Work out the finished part from the listing and answer in its coordinate system (mm). Face numbers are marked on the shaded views. A direction names the side the tool comes from. Give positions to 0.01 mm unless a question says otherwise; leave off trailing zeros. Loops run counter-clockwise (first coordinate to the right, second up) from the corner with the lowest first, then second, coordinate; pieces in that order, holes last. Notation, with made-up numbers: (67.5, -18.5) - (82.5, -18.5) arc R24 cw to (82.5, 20.5) - close; hole circle Ø11 at (-39, -2.75). An arc over 180 degrees is marked (long way). One line per item, written item: value.
Autodesk Inventor part; units mm, degrees
ref_plane "YZ Plane" through (0, 0, 0) normal (1, 0, 0) x (0, 1, 0)
ref_plane "XZ Plane" through (0, 0, 0) normal (0, 1, 0) x (-1, 0, 0)
ref_plane "XY Plane" through (0, 0, 0) normal (0, 0, 1) x (1, 0, 0)
sketch "Sketch1" plane through (0, 0, 0) normal (0, 1, 0) x (-1, 0, 0)
  line L0 (0, 0) -> (200, 0)
  line L1 (200, 0) -> (200, -200)
  line L2 (200, -200) -> (0, -200)
  line L3 (0, -200) -> (0, 0)
  line L4 (198, -198) -> (198, -2)
  line L5 (198, -2) -> (2, -2)
  line L6 (2, -2) -> (2, -198)
  line L7 (2, -198) -> (198, -198)
  dimension "d0" = 200
  dimension "d1" = 200
  dimension "d2" = 2
extrude "Extrusion1" add sketch "Sketch1" against normal blind 65 contours L0 L1 L2 L3 | L7 L6 L5 L4
sketch "Sketch2" plane through (0, 0, 0) normal (0, 1, 0) x (1, 0, 0)
  line L0 (-198.5, 198.5) -> (-1.5, 198.5)
  line L1 (-1.5, 198.5) -> (-1.5, 1.5)
  line L2 (-1.5, 1.5) -> (-198.5, 1.5)
  line L3 (-198.5, 1.5) -> (-198.5, 198.5)
  line L4 (-200, 200) -> (-200, 0)
  line L5 (0, 200) -> (-200, 200)
  line L6 (-109.0225, 121.8048) -> (-59.0225, 121.8048)
  line L7 (-59.0225, 121.8048) -> (-59.0225, 76.8048)
  line L8 (-59.0225, 76.8048) -> (-109.0225, 76.8048)
  line L9 (-109.0225, 76.8048) -> (-109.0225, 121.8048)
  circle A0 centre (-100, 100) radius 4
  point P0 (0, 0)
  dimension "d5" = 197
  dimension "d6" = 197
  dimension "d7" = 1.5
  dimension "d8" = 1.5
  dimension "d37" = 50
  dimension "d38" = 45
  dimension "d39" = 8
extrude "Extrusion2" cut sketch "Sketch2" against normal blind 63 contours L0 L1 L2 L3 | L6 L7 L8 L9 | A0
sketch "Sketch3" plane through (-200, 0, 0) normal (0, 0, 1) x (1, 0, 0)
  line L0 (25, -35) -> (25, -65)
  line L1 (25, -65) -> (175, -65)
  line L2 (175, -65) -> (175, -35)
  line L3 (175, -35) -> (25, -35)
  line L4 (200, 0) -> (200, -65)
  line L5 (42.8625, -63) -> (47.625, -63)
  line L6 (198.5, -63) -> (1.5, -63)
  line L7 (200, -65) -> (0, -65)
  dimension "d11" = 150
  dimension "d12" = 30
  dimension "d13" = 25
  dimension "d14" = 0
  dimension "d36" = 0
extrude "Extrusion3" cut sketch "Sketch3" against normal blind 3
sketch "Sketch4" plane through (0, 0, -200) normal (0, 0, -1) x (-1, 0, 0)
  line L0 (40.0009, -61.5) -> (40.0009, -46.5)
  line L1 (0.0009, -46.5) -> (40.0009, -46.5)
  line L2 (40.0009, -61.5) -> (0.0009, -61.5)
  line L3 (0.0009, -61.5) -> (0.0009, -46.5)
  line L4 (0.0009, -46.5) -> (40.0009, -46.5)
  line L5 (40.0009, -46.5) -> (40.0009, -61.5)
  line L6 (200, -65) -> (0, -65)
  point P0 (48.3834, -59.8808)
  point P1 (40.0009, -54)
  point P2 (0.0009, -54)
  dimension "d27" = 40
  dimension "d28" = 15
  dimension "d29" = 3.5
extrude "Extrusion4" cut sketch "Sketch4" against normal blind 3
sketch "Sketch5" plane through (0, 0, 0) normal (1, 0, 0) x (0, 0, -1)
  line L0 (200, -61.5) -> (160, -61.5)
  line L1 (160, -61.5) -> (160, -46.5)
  line L2 (160, -46.5) -> (200, -46.5)
  line L3 (200, -46.5) -> (200, -61.5)
  point P0 (0, 0)
  point P1 (160, -54)
  dimension "d30" = 40
  dimension "d33" = 15
extrude "Extrusion5" cut sketch "Sketch5" against normal blind 3
ref_plane "Work Plane4" through (-100, -62, -100) normal (0, 1, 0) x (1, 0, 0)
sketch "Sketch7" plane through (-100, -62, -100) normal (0, 1, 0) x (1, 0, 0)
  line L0 (31.2315, 20.7219) -> (-8.7685, 20.7219)
  line L1 (-8.7685, -19.2781) -> (31.2315, -19.2781)
  line L2 (-8.7685, 20.7219) -> (7.9375, 20.7219)
  line L3 (7.9375, 20.7219) -> (7.9375, -19.2781)
  line L4 (7.9375, -19.2781) -> (-8.7685, -19.2781)
  line L5 (-8.7685, -19.2781) -> (-8.7685, 20.7219)
  circle A0 centre (0, 0) radius 3
  point P0 (100, -100)
  dimension "d51" = 6
extrude "Extrusion7" add sketch "Sketch7" along normal blind 39 contours A0
ref_plane "Work Plane3" through (0, -35, 0) normal (0, 1, 0) x (1, 0, 0)
sketch "Sketch9" plane through (-100, -23, -100) normal (0, 1, 0) x (1, 0, 0)
  point P0 (100, -100)
  point P1 (-0.0134, 0.0104)
hole "Hole1" at (-100.0134, -23, -100.0104) direction (0, -1, 0) diameter 2.7 depth 5
sketch "Sketch16" plane through (0, -63, 0) normal (0, 1, 0) x (1, 0, 0)
  line L0 (-183.7981, 135.019) -> (-127.7981, 135.019)
  line L1 (-127.7981, 135.019) -> (-127.7981, 50.019)
  line L2 (-127.7981, 50.019) -> (-183.7981, 50.019)
  line L3 (-183.7981, 50.019) -> (-183.7981, 135.019)
  circle A0 centre (-131.5481, 111.769) radius 2.5
  circle A1 centre (-131.5481, 53.769) radius 2.5
  circle A2 centre (-180.0481, 111.769) radius 2.5
  circle A3 centre (-180.0481, 53.769) radius 2.5
  point P0 (0, 0)
  dimension "d106" = 85
  dimension "d107" = 56
  dimension "d108" = 5
  dimension "d109" = 5
  dimension "d110" = 23.25
  dimension "d111" = 58
  dimension "d112" = 3.75
  dimension "d113" = 5
  dimension "d114" = 5
  dimension "d115" = 58
  dimension "d116" = 23.25
  dimension "d117" = 48.5
  dimension "d118" = 3.75
  dimension "d119" = 3.75
  dimension "d120" = 48.5
extrude "Extrusion14" add sketch "Sketch16" along normal blind 8 contours A0 | A1 | A2 | A3
sketch "Sketch18" plane through (-180.0481, -55, -111.769) normal (0, 1, 0) x (1, 0, 0)
  point P0 (180.0481, -111.769)
  point P1 (0.0125, -0.0104)
hole "Hole4" at (-180.0357, -55, -111.7586) direction (0, -1, 0) diameter 2.6 depth 5
sketch "Sketch19" plane through (-131.5481, -55, -111.769) normal (0, 1, 0) x (1, 0, 0)
  point P0 (131.5481, -111.769)
  point P1 (0.007, -0.059)
hole "Hole5" at (-131.5412, -55, -111.7101) direction (0, -1, 0) diameter 2.6 depth 5
sketch "Sketch20" plane through (-180.0481, -55, -53.769) normal (0, 1, 0) x (1, 0, 0)
  point P0 (180.0481, -53.769)
  point P1 (0.0525, -0.0221)
hole "Hole6" at (-179.9956, -55, -53.747) direction (0, -1, 0) diameter 2.6 depth 5
sketch "Sketch21" plane through (-131.5481, -55, -53.769) normal (0, 1, 0) x (1, 0, 0)
  point P0 (131.5481, -53.769)
  point P1 (0.0019, 0.0101)
hole "Hole7" at (-131.5462, -55, -53.7792) direction (0, -1, 0) diameter 2.6 depth 5
sketch "Sketch23" plane through (-200, 0, 0) normal (0, 0, 1) x (1, 0, 0)
  line L0 (200, 0) -> (200, -65)
  line L1 (-0.0001, 0) -> (200, 0)
  line L2 (200, 0) -> (200, -21)
  line L3 (200, -21) -> (-0.0001, -21)
  line L4 (-0.0001, -21) -> (-0.0001, 0)
  dimension "d158" = 21
extrude "Extrusion15" cut sketch "Sketch23" against normal blind 3
sketch "Sketch24" plane through (0, -65, 0) normal (1, 0, 0) x (0, 0, -1)
  line L0 (2.6301, 65) -> (209.4801, 65)
  line L1 (209.4801, 65) -> (209.4801, 44)
  line L2 (209.4801, 44) -> (2.6301, 44)
  line L3 (2.6301, 44) -> (2.6301, 65)
  point P0 (0, 65)
  point P1 (-254.0504, -31.9889)
  dimension "d161" = 21
extrude "Extrusion16" cut sketch "Sketch24" against normal blind 1.5
sketch "Sketch25" plane through (0, -65, -200) normal (0, 0, -1) x (-1, 0, 0)
  line L0 (198.5, 65) -> (1.5, 65)
  line L1 (1.5, 65) -> (200, 65)
  line L2 (200, 65) -> (200, 44)
  line L3 (200, 44) -> (1.5, 44)
  line L4 (1.5, 44) -> (1.5, 65)
  point P0 (0, 65)
  dimension "d164" = 21
extrude "Extrusion17" cut sketch "Sketch25" against normal blind 1.5
sketch "Sketch29" plane through (0, -63, 0) normal (0, 1, 0) x (1, 0, 0)
  circle A0 centre (-87.6204, 99.9966) radius 2.4
  circle A1 centre (-100.007, 99.1404) radius 1.5875
  line L0 (-81.6277, 78.5588) -> (-81.6277, 83.3088)
  line L1 (-81.6277, 83.3088) -> (-93.6277, 83.3088)
  line L2 (-93.6277, 83.3088) -> (-93.6277, 78.5588)
  line L3 (-93.6277, 83.3088) -> (-81.6132, 83.3088)
  line L4 (-81.6132, 83.3088) -> (-81.6132, 106.3088)
  line L5 (-81.6132, 106.3088) -> (-93.6277, 106.3088)
  line L6 (-93.6277, 106.3088) -> (-93.6277, 83.3088)
  line L7 (-93.6277, 106.3088) -> (-81.6132, 106.3088)
  line L8 (-81.6132, 106.3088) -> (-81.6132, 111.0588)
  line L9 (-93.6277, 111.0588) -> (-93.6277, 106.3088)
  arc A2 (-87.2339, 79.8817) -> (-88.0214, 79.8817) centre (-87.6277, 80.9088) ccw
  arc A3 (-87.9871, 109.7433) -> (-87.2394, 109.7433) centre (-87.6132, 108.7088) ccw
  line L10 (-88.0214, 79.8817) -> (-88.0068, 79.8817)
  line L11 (-88.0068, 78.5588) -> (-88.0214, 78.5588)
  line L12 (-88.0214, 78.5588) -> (-88.0214, 79.8817)
  line L13 (-88.0214, 79.8817) -> (-88.0068, 79.8817)
  line L14 (-88.0068, 78.5588) -> (-88.0214, 78.5588)
  line L15 (-88.0214, 78.5588) -> (-88.0214, 79.8817)
  line L16 (-148.191, 49.2124) -> (-151.9502, 49.2124)
  line L17 (-87.2339, 79.8817) -> (-87.2339, 78.5588)
  line L18 (-88.0068, 109.7433) -> (-88.0068, 111.0662)
  line L19 (-88.0068, 109.7433) -> (-88.0068, 111.0662)
  line L20 (-87.613, 87.7328) -> (-87.613, 87.7254)
  line L21 (-87.2193, 111.0662) -> (-87.2193, 109.7433)
  line L22 (-87.9871, 109.7433) -> (-88.0068, 109.7433)
  line L23 (-87.9871, 109.7433) -> (-88.0068, 109.7433)
  line L24 (-87.2193, 109.7433) -> (-87.2394, 109.7433)
  line L25 (-87.2339, 111.0662) -> (-87.2193, 111.0662)
  circle A4 centre (-87.6132, 100.0088) radius 2.4
  circle A5 centre (-87.6132, 100.0088) radius 5.7525
  line L26 (-93.6277, 78.5588) -> (-88.0214, 78.5588)
  line L27 (-87.2339, 78.5588) -> (-81.6277, 78.5588)
  line L28 (-81.6132, 111.0588) -> (-87.2193, 111.0588)
  line L29 (-88.0068, 111.0588) -> (-93.6277, 111.0588)
  circle A6 centre (-87.6277, 80.9088) radius 1.75
  circle A7 centre (-87.6132, 108.7088) radius 1.75
  point P0 (0, 0)
  point P1 (-365.9025, -227.0891)
  point P2 (-350.612, -204.1468)
  point P3 (-350.6265, -227.1468)
  point P4 (-145.8741, 48.5842)
  dimension "d178" = 12.3867
  dimension "d186" = 12
  dimension "d187" = 4.75
  dimension "d188" = 23
  dimension "d189" = 4.75
  dimension "d190" = 2.2
  dimension "d191" = 2.2
  dimension "d192" = -27.8
  dimension "d193" = 4.8
  dimension "d196" = 3.5
  dimension "d197" = 3.5
sketch "Sketch30" plane through (0, -63, 0) normal (0, 1, 0) x (1, 0, 0)
  line L0 (-108.5304, 108.0352) -> (-93.5304, 108.0352)
  line L1 (-93.5304, 108.0352) -> (-93.5304, 93.0352)
  line L2 (-93.5304, 93.0352) -> (-108.5304, 93.0352)
  line L3 (-108.5304, 93.0352) -> (-108.5304, 108.0352)
  point P0 (0, 0)
  dimension "d171" = 15
  dimension "d172" = 15
extrude "Extrusion19" add sketch "Sketch30" along normal blind 20
sketch "Sketch31" plane through (-200, -65, -200) normal (-1, 0, 0) x (0, 0, 1)
  point P0 (200, 65)
sketch "Sketch32" plane through (-200, -65, -200) normal (-1, 0, 0) x (0, 0, 1)
  line L0 (1.5, 65) -> (0, 65)
  line L1 (0, 65) -> (197, 65)
  line L2 (197, 65) -> (197, 44)
  line L3 (197, 44) -> (0, 44)
  line L4 (0, 44) -> (0, 65)
  point P0 (200, 65)
extrude "Extrusion20" cut sketch "Sketch32" against normal blind 1.5
sketch "Sketch34" plane through (0, -63, 0) normal (0, 1, 0) x (1, 0, 0)
  line L0 (-93.5304, 106.9186) -> (-77.5304, 106.9186)
  line L1 (-77.5304, 106.9186) -> (-77.5304, 106.4186)
  line L2 (-77.5304, 106.4186) -> (-93.5304, 106.4186)
  line L3 (-93.5304, 106.4186) -> (-93.5304, 106.9186)
  line L4 (-93.9801, 83.2121) -> (-77.9801, 83.2121)
  line L5 (-77.9801, 83.2121) -> (-77.9801, 82.7121)
  line L6 (-77.9801, 82.7121) -> (-93.9801, 82.7121)
  line L7 (-93.9801, 82.7121) -> (-93.9801, 83.2121)
  point P0 (0, 0)
  dimension "d179" = 16
  dimension "d180" = 0.5
  dimension "d181" = 16
  dimension "d182" = 0.5
extrude "Extrusion21" add sketch "Sketch34" along normal blind 1
extrude "Extrusion22" add sketch "Sketch29" along normal blind 17.3 contours A6 L12 A2 L17 | L17 A2 L12 A6 | A7 L21 L24 A3 L22 L18 | L18 L22 A3 L24 L21 A7
sketch "Sketch35" plane through (-87.6132, -45.7, -108.7088) normal (0, 1, 0) x (1, 0, 0)
  circle A0 centre (0, 0) radius 1
  circle A1 centre (0, -27.804) radius 1
  point P0 (87.6132, -108.7088)
  dimension "d200" = 2
  dimension "d201" = 2
hole "Hole8" at (-87.6132, -45.7, -108.7088) at (-87.6132, -45.7, -80.9048) direction (0, -1, 0) diameter 2 depth 30
sketch "Sketch36" plane through (0, -63, 0) normal (0, 1, 0) x (1, 0, 0)
  line L0 (-77.5304, 106.9186) -> (-93.5304, 106.9186)
  line L1 (-93.2842, 110.9186) -> (-82.1811, 110.9186)
  line L2 (-82.1811, 110.9186) -> (-82.1811, 106.9186)
  line L3 (-82.1811, 106.9186) -> (-93.2842, 106.9186)
  line L4 (-93.2842, 106.9186) -> (-93.2842, 110.9186)
  point P0 (0, 0)
  dimension "d212" = 4
extrude "Extrusion23" add sketch "Sketch36" along normal blind 10
sketch "Sketch37" plane through (-82.1811, -63, -110.9186) normal (0, 0, -1) x (-1, 0, 0)
  line L0 (1.5875, 8.0595) -> (9.525, 8.0595)
  line L1 (9.525, 8.0595) -> (9.525, 0.0595)
  line L2 (9.525, 0.0595) -> (1.5875, 0.0595)
  line L3 (1.5875, 0.0595) -> (1.5875, 8.0595)
  point P0 (-82.1811, 63)
  dimension "d211" = 8
extrude "Extrusion24" cut sketch "Sketch37" against normal blind 4
properties part number "Box"
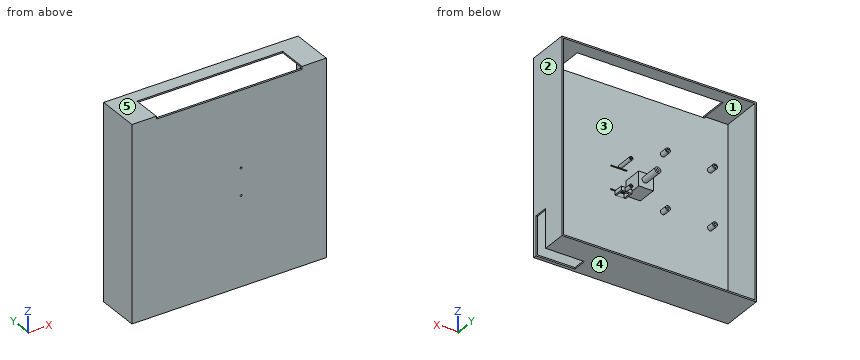
1. Find the intervals of material crossed by line 1 along X through (y, z) = (-53, -106); line 2 along Z through (x, y) = (-79.5, -25.5), in increasing order.
Output:
line 1: x = -200 to -198.5, -108.53 to -93.53, -1.5 to 0
line 2: z = -200 to -198.5, -1.5 to 0
2. Section B-B (x = -139.5) is taken. Write down the section's boundary in (y, z), and give its area (3 significant figures).
Output:
outline: (-65, -200) - (-21, -200) - (-21, -198.5) - (-63, -198.5) - (-63, -3) - (-65, -3) - close; (-35, -1.5) - (-21, -1.5) - (-21, 0) - (-35, 0) - close
area: 478 mm²
3. Section C-C (z = -47) is taken. Write down the section's boundary in (x, y).
Output:
outline: (-200, -65) - (0, -65) - (0, -21) - (-1.5, -21) - (-1.5, -63) - (-198.5, -63) - (-198.5, -21) - (-200, -21) - close
4. Flat-ended cylindrical pins translate along their axes: pin 1 Ø2 at (x, z) = (-139, -84) entering from +Y; pin 2 Ø4.5 at (x, y) = (-85, -58.5) entering from +Z; pin 3 Ø1.2 at (x, z) = (-85.5, -108.5) entering from +Y. Find the tip coordinate at first contact, or state that the pin passes through.
Output:
pin 1: stops at y = -63
pin 2: stops at z = -79.2
pin 3: stops at y = -45.7
5. The mould has two halves that part along Z. Classify the marked faces 3, 4 and 5: released by +Z, released by -Z, zero draft, split by the parting line, or undercut.
Output:
face 3: undercut
face 4: released by -Z
face 5: released by +Z
6. Section A-A (y = -38.5) is taken. Write down the section's boundary in (x, z).
Output:
outline: (-200, -200) - (0, -200) - (0, 0) - (-25, 0) - (-25, -1.5) - (-1.5, -1.5) - (-1.5, -198.5) - (-198.5, -198.5) - (-198.5, -1.5) - (-175, -1.5) - (-175, 0) - (-200, 0) - close; circle Ø6 at (-100, -100)
7. For the marked faces 1 and 2, determine the directions among +Z, -Z, +X, -X, +Y, -Y from which every point of the face is accessible in a straight line to the end or side of a thin tool.
Output:
face 1: +Y
face 2: +Z, -Z, +X, +Y, -Y
